Read the model definition and answer for the solid it produces. Units are mm, in the model's axes. Give positions to 0.01 mm unless a question says otherwise; leave off trailing zeros. Return JSON: item names as keys, results as strings. Group by question number.
from build123d import *

# Parameters (mm, degrees)
F0_R     = 2.1
F1_DEPTH = 1000


# Not quite as in the source:
# - ends of sketch curves that miss each other by under 0.0002 mm in the source are joined


with BuildPart() as f1:
    # F0 (on Top) → F1 (new body)
    with BuildSketch(Plane.XY):
        with BuildLine():
            Line((-2.860219, 3.085333), (-2.860219, 5.198566))
            ThreePointArc((-2.860219, 5.198566), (-2.7720364303, 5.4101211696), (-2.56022, 5.497674))
            Line((-2.56022, 5.497674), (-1.22022, 5.497674))
            Line((-1.22022, 5.497674), (1.349586, 2.927868))
            ThreePointArc((1.349586, 2.927868), (1.4146178598, 2.8305410297), (1.437454, 2.715736))
            Line((1.437454, 2.715736), (1.437454, 0.1))
            Line((1.437454, 0.1), (1.637454, 0))
            Line((1.637454, 0), (1.437454, -0.1))
            Line((1.437454, -0.1), (1.437454, -2.715736))
            ThreePointArc((1.437454, -2.715736), (1.4146178598, -2.8305410297), (1.3495860344, -2.9278680344))
            Line((1.3495860344, -2.9278680344), (-1.22022, -5.497674))
            Line((-1.22022, -5.497674), (-2.56022, -5.497674))
            ThreePointArc((-2.56022, -5.497674), (-2.7720364303, -5.4101211696), (-2.8602186739, -5.198565999))
            Line((-2.8602186739, -5.198565999), (-2.860219, -3.085333))
            Line((-2.860219, -3.085333), (-4.661886, -4.887))
            Line((-4.661886, -4.887), (-4.661886, -9.6))
            ThreePointArc((-4.661886, -9.6), (-4.5447287125, -9.8828427125), (-4.261886, -10))
            Line((-4.261886, -10), (0.451114, -10))
            Line((0.451114, -10), (2.252781, -8.198333))
            Line((2.252781, -8.198333), (0.139548, -8.198333))
            ThreePointArc((0.139548, -8.198333), (-0.0720071696, -8.1101504303), (-0.15956, -7.898334))
            Line((-0.15956, -7.898334), (-0.15956, -6.558334))
            Line((-0.15956, -6.558334), (2.410246, -3.988528))
            ThreePointArc((2.410246, -3.988528), (2.5075729703, -3.9234961402), (2.622378, -3.90066))
            Line((2.622378, -3.90066), (5.238114, -3.90066))
            Line((5.238114, -3.90066), (5.338114, -3.70066))
            Line((5.338114, -3.70066), (5.438114, -3.90066))
            Line((5.438114, -3.90066), (8.05385, -3.90066))
            ThreePointArc((8.05385, -3.90066), (8.1686550297, -3.9234961402), (8.2659820344, -3.9885279656))
            Line((8.2659820344, -3.9885279656), (10.835788, -6.558334))
            Line((10.835788, -6.558334), (10.835788, -7.898334))
            ThreePointArc((10.835788, -7.898334), (10.7482351696, -8.1101504303), (10.536679999, -8.1983326739))
            Line((10.536679999, -8.1983326739), (8.423447, -8.198333))
            Line((8.423447, -8.198333), (10.225114, -10))
            Line((10.225114, -10), (20.451114, -10))
            Line((20.451114, -10), (22.252781, -8.198333))
            Line((22.252781, -8.198333), (20.139548, -8.198333))
            ThreePointArc((20.139548, -8.198333), (19.9279928304, -8.1101504303), (19.84044, -7.898334))
            Line((19.84044, -7.898334), (19.84044, -6.558334))
            Line((19.84044, -6.558334), (22.410246, -3.988528))
            ThreePointArc((22.410246, -3.988528), (22.5075729703, -3.9234961402), (22.622378, -3.90066))
            Line((22.622378, -3.90066), (25.238114, -3.90066))
            Line((25.238114, -3.90066), (25.338114, -3.70066))
            Line((25.338114, -3.70066), (25.438114, -3.90066))
            Line((25.438114, -3.90066), (28.05385, -3.90066))
            ThreePointArc((28.05385, -3.90066), (28.1686550297, -3.9234961402), (28.2659820344, -3.9885279656))
            Line((28.2659820344, -3.9885279656), (30.835788, -6.558334))
            Line((30.835788, -6.558334), (30.835788, -7.898334))
            ThreePointArc((30.835788, -7.898334), (30.7482351696, -8.1101504303), (30.536679999, -8.1983326739))
            Line((30.536679999, -8.1983326739), (28.423447, -8.198333))
            Line((28.423447, -8.198333), (30.225114, -10))
            Line((30.225114, -10), (34.938114, -10))
            ThreePointArc((34.938114, -10), (35.2209567125, -9.8828427125), (35.338114, -9.6))
            Line((35.338114, -9.6), (35.338114, -4.887))
            Line((35.338114, -4.887), (33.536447, -3.085333))
            Line((33.536447, -3.085333), (33.536447, -5.198566))
            ThreePointArc((33.536447, -5.198566), (33.4482644303, -5.4101211696), (33.236448, -5.497674))
            Line((33.236448, -5.497674), (31.896448, -5.497674))
            Line((31.896448, -5.497674), (29.326642, -2.927868))
            ThreePointArc((29.326642, -2.927868), (29.2616101402, -2.8305410297), (29.238774, -2.715736))
            Line((29.238774, -2.715736), (29.238774, -0.1))
            Line((29.238774, -0.1), (29.038774, 0))
            Line((29.038774, 0), (29.238774, 0.1))
            Line((29.238774, 0.1), (29.238774, 2.715736))
            ThreePointArc((29.238774, 2.715736), (29.2616101402, 2.8305410297), (29.3266419656, 2.9278680344))
            Line((29.3266419656, 2.9278680344), (31.896448, 5.497674))
            Line((31.896448, 5.497674), (33.236448, 5.497674))
            ThreePointArc((33.236448, 5.497674), (33.4482644303, 5.4101211696), (33.5364466739, 5.198565999))
            Line((33.5364466739, 5.198565999), (33.536447, 3.085333))
            Line((33.536447, 3.085333), (35.338114, 4.887))
            Line((35.338114, 4.887), (35.338114, 9.6))
            ThreePointArc((35.338114, 9.6), (35.2209567125, 9.8828427125), (34.938114, 10))
            Line((34.938114, 10), (30.225114, 10))
            Line((30.225114, 10), (28.423447, 8.198333))
            Line((28.423447, 8.198333), (30.53668, 8.198333))
            ThreePointArc((30.53668, 8.198333), (30.7482351696, 8.1101504303), (30.835788, 7.898334))
            Line((30.835788, 7.898334), (30.835788, 6.558334))
            Line((30.835788, 6.558334), (28.265982, 3.988528))
            ThreePointArc((28.265982, 3.988528), (28.1686550297, 3.9234961402), (28.05385, 3.90066))
            Line((28.05385, 3.90066), (25.438114, 3.90066))
            Line((25.438114, 3.90066), (25.338114, 3.70066))
            Line((25.338114, 3.70066), (25.238114, 3.90066))
            Line((25.238114, 3.90066), (22.622378, 3.90066))
            ThreePointArc((22.622378, 3.90066), (22.5075729703, 3.9234961402), (22.4102459656, 3.9885279656))
            Line((22.4102459656, 3.9885279656), (19.84044, 6.558334))
            Line((19.84044, 6.558334), (19.84044, 7.898334))
            ThreePointArc((19.84044, 7.898334), (19.9279928304, 8.1101504303), (20.139548001, 8.1983326739))
            Line((20.139548001, 8.1983326739), (22.252781, 8.198333))
            Line((22.252781, 8.198333), (20.451114, 10))
            Line((20.451114, 10), (10.225114, 10))
            Line((10.225114, 10), (8.423447, 8.198333))
            Line((8.423447, 8.198333), (10.53668, 8.198333))
            ThreePointArc((10.53668, 8.198333), (10.7482351696, 8.1101504303), (10.835788, 7.898334))
            Line((10.835788, 7.898334), (10.835788, 6.558334))
            Line((10.835788, 6.558334), (8.265982, 3.988528))
            ThreePointArc((8.265982, 3.988528), (8.1686550297, 3.9234961402), (8.05385, 3.90066))
            Line((8.05385, 3.90066), (5.438114, 3.90066))
            Line((5.438114, 3.90066), (5.338114, 3.70066))
            Line((5.338114, 3.70066), (5.238114, 3.90066))
            Line((5.238114, 3.90066), (2.622378, 3.90066))
            ThreePointArc((2.622378, 3.90066), (2.5075729703, 3.9234961402), (2.4102459656, 3.9885279656))
            Line((2.4102459656, 3.9885279656), (-0.15956, 6.558334))
            Line((-0.15956, 6.558334), (-0.15956, 7.898334))
            ThreePointArc((-0.15956, 7.898334), (-0.0720071696, 8.1101504303), (0.139548001, 8.1983326739))
            Line((0.139548001, 8.1983326739), (2.252781, 8.198333))
            Line((2.252781, 8.198333), (0.451114, 10))
            Line((0.451114, 10), (-4.261886, 10))
            ThreePointArc((-4.261886, 10), (-4.5447287125, 9.8828427125), (-4.661886, 9.6))
            Line((-4.661886, 9.6), (-4.661886, 4.887))
            Line((-4.661886, 4.887), (-2.860219, 3.085333))
        make_face()
        with Locations((5.338114, 0)):
            Circle(F0_R, mode=Mode.SUBTRACT)
        Polygon((12.638114, 6.24), (12.638114, 8.2), (18.038114, 8.2), (18.038114, 6.24), (21.349586, 2.927868), (21.437454, 2.715736), (21.437454, 0.1), (21.637454, 0), (21.437454, -0.1), (21.437454, -2.715736), (21.267706, -3.009748), (18.038114, -6.24), (18.037784, -8.2), (12.638114, -8.2), (12.638444, -6.23967), (9.326642, -2.927868), (9.238774, -2.715736), (9.238774, -0.1), (9.038774, 0), (9.238774, 0.1), (9.238774, 2.715736), (9.326642, 2.927868), align=None, mode=Mode.SUBTRACT)
        with Locations((25.338114, 0)):
            Circle(F0_R, mode=Mode.SUBTRACT)
    extrude(amount=F1_DEPTH)


solid = f1.part
1. Straight lines are drawn through the part: line 1 (X direction, y = -0.5, z = 520.5); line 2 (Y direction, x = 10.5, z = 575); line 3 (X direction, y = -7.5, z = 790). For each, find the intervals that lie inside material, in ascending order. Write a range as from..to.
2. Flat-ended cylindrical pins translate along their axes: pin 1 Ø2 at (x, y) = (1.5, 6.5) entering from +Z; pin 2 Ø3 at (x, z) = (26.5, 654) entering from -Y; pin 3 Ø1.3 at (x, z) = (7, 543) entering from +Y; pin 4 Ø3 at (y, z) = (1, 662.5) entering from -X. Find the tip coordinate at first contact, or state that the pin passes through.
3. Section A-A on z = 503.5 is taken. State how many separate pieces and enclosed holes the cut face has, then the cut area to 3 significant figures.
Completed:
{
 "1": {"line 1": "x = 1.44..3.3, 7.38..9.24, 21.44..23.3, 27.38..29.24", "line 2": "y = -10..-8.2, -6.22..-4.1, 4.1..6.22, 8.2..10", "line 3": "x = -4.66..-0.16, 10.84..12.64, 18.04..19.84, 30.84..35.34"},
 "2": {"pin 1": "passes through", "pin 2": "stops at y = -3.9", "pin 3": "stops at y = 3.9", "pin 4": "stops at x = 1.44"},
 "3": {"separate pieces": "1", "enclosed holes": "3", "area": "295 mm²"}
}
